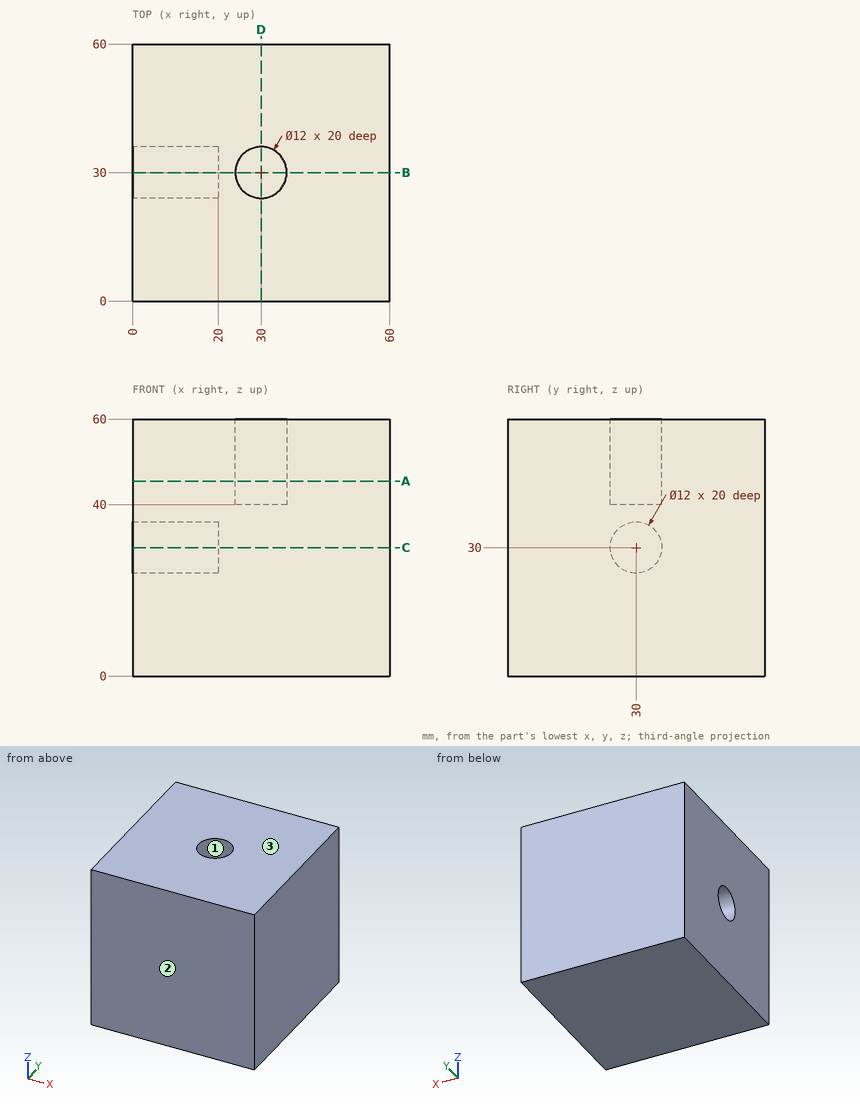
Verification items for this drawing (mm, ordinates from the low corner). Coordinates: 2 decimals unless noted, no trailing zeros. Loops run counter-clockwise (first coordinate to the right, second up) from the corner with the lowest first, then second, coordinate; pieces in that order, holes last. Notation, with made-up numbers: (67.5, 37.5) -> (106.5, 37.5) arc R15 ccw to (106.5, 46.5) -> close; hole circle Ø2 at (-13.5, 41.5). An arc over 180 degrees is marked (long way). Answer in a Markdown table with one row per item. Add a question column.
1. Section check B-B, the plane y = 30. Enter the section's corners in (x, z).
2. Section check A-A, the plane z = 45.5. Enter the section's corners in (x, y), then the cut area to 3 significant figures.
3. Section check C-C, the plane z = 30. Enter the section's corners in (x, y).
4. Draft check along Y on the marked faces 1, 2 and 3. Enter one of: +Y half, -Y half, draft (parallel to the pull), parting line (faces both ways), or undercut.
5. Section check D-D, the plane x = 30. Enter the section's corners in (y, z), then the cut area to 3 significant figures.
6. Material ranges on probe 1 along Y at (x, z) = (15.75, 30); probe 2 along Z at (x, y) = (8, 31.5); probe 3 along X at (y, z) = (32, 50.5), recorded low to high. Write a range as [from, to].
7. Depth check by flat-ended pin: P1, Ø9.5, axis at x = 30, y = 30, coming from the +Z side. Enter the tip coordinate at first touch or a pass-through.
Derived:
| question | item | result |
|---|---|---|
| 1 | outline | (0, 0) -> (60, 0) -> (60, 60) -> (36, 60) -> (36, 40) -> (24, 40) -> (24, 60) -> (0, 60) -> (0, 36) -> (20, 36) -> (20, 24) -> (0, 24) -> close |
| 2 | outline | (0, 0) -> (60, 0) -> (60, 60) -> (0, 60) -> close; hole circle Ø12 at (30, 30) |
| 2 | area | 3,490 mm² |
| 3 | outline | (0, 0) -> (60, 0) -> (60, 60) -> (0, 60) -> (0, 36) -> (20, 36) -> (20, 24) -> (0, 24) -> close |
| 4 | face 1 | undercut |
| 4 | face 2 | -Y half |
| 4 | face 3 | draft |
| 5 | outline | (0, 0) -> (60, 0) -> (60, 60) -> (36, 60) -> (36, 40) -> (24, 40) -> (24, 60) -> (0, 60) -> close |
| 5 | area | 3,360 mm² |
| 6 | probe 1 | y = [0, 24], [36, 60] |
| 6 | probe 2 | z = [0, 24.19], [35.81, 60] |
| 6 | probe 3 | x = [0, 24.34], [35.66, 60] |
| 7 | P1 | stops at z = 40 |
